Build history of the part. All positions in model axes, mm. Face numbers are marked on the shaded views. A direction names the side the tool comes from. Round coordinates to 2 decimals unless told otherwise and drop trailing zeros. Loops run counter-clockwise (first coordinate to the right, second up) from the corner with the lowest first, then second, coordinate; pieces in that order, holes last. Notation, with made-up numbers: M -25.5,-34 L 3.5,-34 A8 ccw 3.5,-22 Z; hole C 26.5,24.5 d3. An arc over 180 degrees is marked long. One line per item, written item: value.
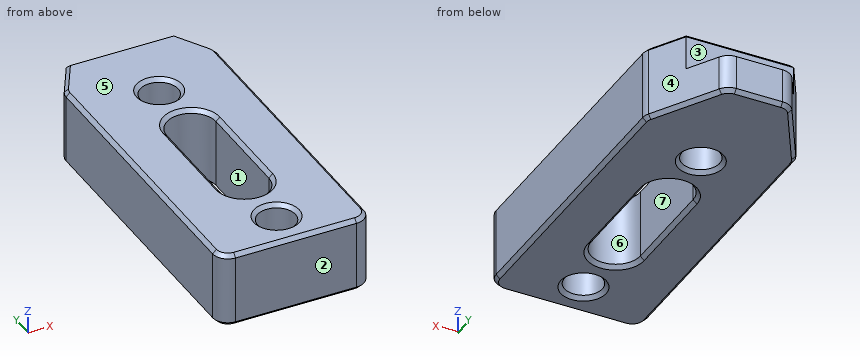
Autodesk Fusion 360 part; units mm, degrees
sketch "Skizze1" plane through (0, 0, 0) normal (0, 0, 1) x (1, 0, 0)
  line L0 (2, 0) -> (18, 0)
  line L1 (20, 2) -> (20, 39.4641)
  line L2 (13.0718, 50) -> (6.9282, 50)
  line L3 (0, 39.4641) -> (0, 2)
  line L4 (10, 50) -> (10, 0) construction
  circle A0 centre (10, 5) radius 2.5
  circle A1 centre (10, 35) radius 2.5
  line L5 (13.25, 26.75) -> (13.25, 13.25)
  line L6 (6.75, 13.25) -> (6.75, 26.75)
  arc A2 (13.25, 26.75) -> (6.75, 26.75) centre (10, 26.75) ccw
  arc A3 (6.75, 13.25) -> (13.25, 13.25) centre (10, 13.25) ccw
  line L7 (0, 40) -> (20, 40) construction
  line L8 (0.2679, 40.4641) -> (5.1962, 49)
  line L9 (19.7321, 40.4641) -> (14.8038, 49)
  line L10 (0, 45) -> (20, 45) construction
  line L11 (0, 26.75) -> (20, 26.75) construction
  line L12 (0, 13.25) -> (20, 13.25) construction
  line L13 (2.8868, 45) -> (17.1132, 45)
  arc A4 (0, 2) -> (2, 0) centre (2, 2) ccw
  arc A5 (18, 0) -> (20, 2) centre (18, 2) ccw
  arc A6 (0.2679, 40.4641) -> (0, 39.4641) centre (2, 39.4641) ccw
  arc A7 (20, 39.4641) -> (19.7321, 40.4641) centre (18, 39.4641) ccw
  arc A8 (14.8038, 49) -> (13.0718, 50) centre (13.0718, 48) ccw
  arc A9 (6.9282, 50) -> (5.1962, 49) centre (6.9282, 48) ccw
  point P0 (20, 0)
  point P1 (20, 40)
  dimension "breite" = 20
  dimension "loch_durchmesser" = 5
  dimension "d4" = 20
  dimension "d6" = 5
  dimension "d7" = 5
  dimension "d8" = 5
  dimension "d9" = 8.25
  dimension "d10" = 8.25
  dimension "kopf_lenge" = 10
  dimension "d13" = 10
  dimension "d14" = 60
  dimension "d15" = 60
  dimension "kopf_winkel" = 60
  dimension "d18" = 5
  dimension "d19" = 6.5
  dimension "d21" = 5
  dimension "d22" = 50
  dimension "d23" = 10
  dimension "d24" = 5
  dimension "parameter_1" = 2.5
  dimension "abrundung" = 2
  dimension "d27" = 2
  dimension "d28" = 2
  dimension "d29" = 2
  dimension "d30" = 2
  dimension "d31" = 2
  dimension "d32" = 2
extrude "Extrusion1" add sketch "Skizze1" against normal blind 10
extrude "Extrusion2" cut sketch "Skizze1" against normal blind 5 contours L2 L8 L9 L13 A8 A9
chamfer "Fase1" distance 0.5 angle 45 34 edges at (10, 30, 0) (13.25, 20, 0) (10, 10, 0) (6.75, 20, 0) (7.6692, 35.904, 0) (7.6692, 5.904, 0) (0, 20.7321, 0) (0.5858, 0.5858, 0) (10, 0, 0) (19.4142, 0.5858, 0) (20, 20.7321, 0) (19.9319, 39.9817, 0) (18.4226, 42.7321, 0) (1.5774, 42.7321, 0) (0.0681, 39.9817, 0) (10, 45, 0) (0, 20.7321, -10) (0.0681, 39.9817, -10) (2.7321, 44.7321, -10) (5.9282, 49.7321, -10) (10, 50, -10) (14.0718, 49.7321, -10) (17.2679, 44.7321, -10) (19.9319, 39.9817, -10) (20, 20.7321, -10) (19.4142, 0.5858, -10) (10, 0, -10) (0.5858, 0.5858, -10) (7.6692, 4.096, -10) (6.75, 20, -10) (10, 10, -10) (13.25, 20, -10) (10, 30, -10) (7.6692, 34.096, -10)
equation "d4 = breite"
equation "d6 = loch_durchmesser"
equation "d7 = loch_durchmesser"
equation "d8 = parameter_1 + loch_durchmesser / 2"
equation "d9 = Linear Dimension-5"
equation "d10 = Linear Dimension-6"
equation "d13 = kopf_lenge"
equation "d14 = kopf_winkel"
equation "d15 = kopf_winkel"
equation "d18 = kopf_lenge / 2"
equation "d19 = Linear Dimension-10"
equation "d21 = kopf_lenge / 2"
equation "d22 = Linear Dimension-11"
equation "d23 = breite / 2"
equation "d24 = parameter_1 + loch_durchmesser / 2"
equation "d27 = abrundung"
equation "d28 = abrundung"
equation "d29 = abrundung"
equation "d30 = abrundung"
equation "d31 = abrundung"
equation "d32 = abrundung"
Item 1: Slice it at C-C, the plane z = -6.5. Give the cut face in (x, y).
Check values:
outline: M 0,2 A2 ccw 2,0 L 18,0 A2 ccw 20,2 L 20,39.46 A2 ccw 19.73,40.46 L 14.8,49 A2 ccw 13.07,50 L 6.93,50 A2 ccw 5.2,49 L 0.27,40.46 A2 ccw 0,39.46 Z; hole M 6.75,13.25 A3.25 ccw 13.25,13.25 L 13.25,26.75 A3.25 ccw 6.75,26.75 Z; hole C 10,5 d5; hole C 10,35 d5
Item 2: Pull direction X, two halves, no side cores. Call the marked faces 4, 5, 6 and 7: pulls with the +X half, pulls with the -X half, needs draft (parallel to the pull), parting line crosses it, or undercut.
Check values:
face 4: pulls with the +X half
face 5: needs draft
face 6: undercut
face 7: undercut
Item 3: Slice it at B-B, the plane x = 10. Give the number of separate pieces and of enclosed holes in the cut face, and give its area (3 significant figures).
Check values:
separate pieces: 4
enclosed holes: 0
area: 173 mm2
Item 4: Drop flat-ended pins along their axis: P1, Ø6.5, axis at x = 10, y = 35, coming from the -Z side; P2, Ø3.5, axis at x = 7.5, z = -3, coming from the +Y side. Give the stop position or say it passes through.
Check values:
P1: stops at z = -10
P2: stops at y = 45
Item 5: Slice it at D-D, the plane z = -4.25. Give the cut face in (x, y), and give its area (3 significant figures).
Check values:
outline: M 0,2 A2 ccw 2,0 L 18,0 A2 ccw 20,2 L 20,39.46 A2 ccw 19.73,40.46 L 17.11,45 L 2.89,45 L 0.27,40.46 A2 ccw 0,39.46 Z; hole M 6.75,13.25 A3.25 ccw 13.25,13.25 L 13.25,26.75 A3.25 ccw 6.75,26.75 Z; hole C 10,5 d5; hole C 10,35 d5
area: 724 mm2
Item 6: Slice it at A-A, the plane y = 24. Give the cut face in (x, z), and give its area (3 significant figures).
Check values:
outline: M 0,-9.5 L 0.5,-10 L 6.25,-10 L 6.75,-9.5 L 6.75,-0.5 L 6.25,0 L 0.5,0 L 0,-0.5 Z; M 13.25,-9.5 L 13.75,-10 L 19.5,-10 L 20,-9.5 L 20,-0.5 L 19.5,0 L 13.75,0 L 13.25,-0.5 Z
area: 134 mm2
Item 7: Wall check: line 1 along Y through (x, z) = (10, -6); line 2 along X through (y, z) = (13, -3.25); line 3 along Y through (x, z) = (9, -4.75). Give the ranges that are in metal, low to high.
Check values:
line 1: y = 0 to 2.5, 7.5 to 10, 30 to 32.5, 37.5 to 50
line 2: x = 0 to 6.76, 13.24 to 20
line 3: y = 0 to 2.71, 7.29 to 10.16, 29.84 to 32.71, 37.29 to 45
Item 8: Which spindle directions (+Z, -Z, +X, -X, +Y, -Y) get a long thin tool onto all of the face, cutting with end or side? Do the marked faces 1, 2 and 3. Say none if no direction does.
Check values:
face 1: +Z, -Z
face 2: +Z, -Z, +X, -X, -Y
face 3: +Z, +X, -X, +Y
